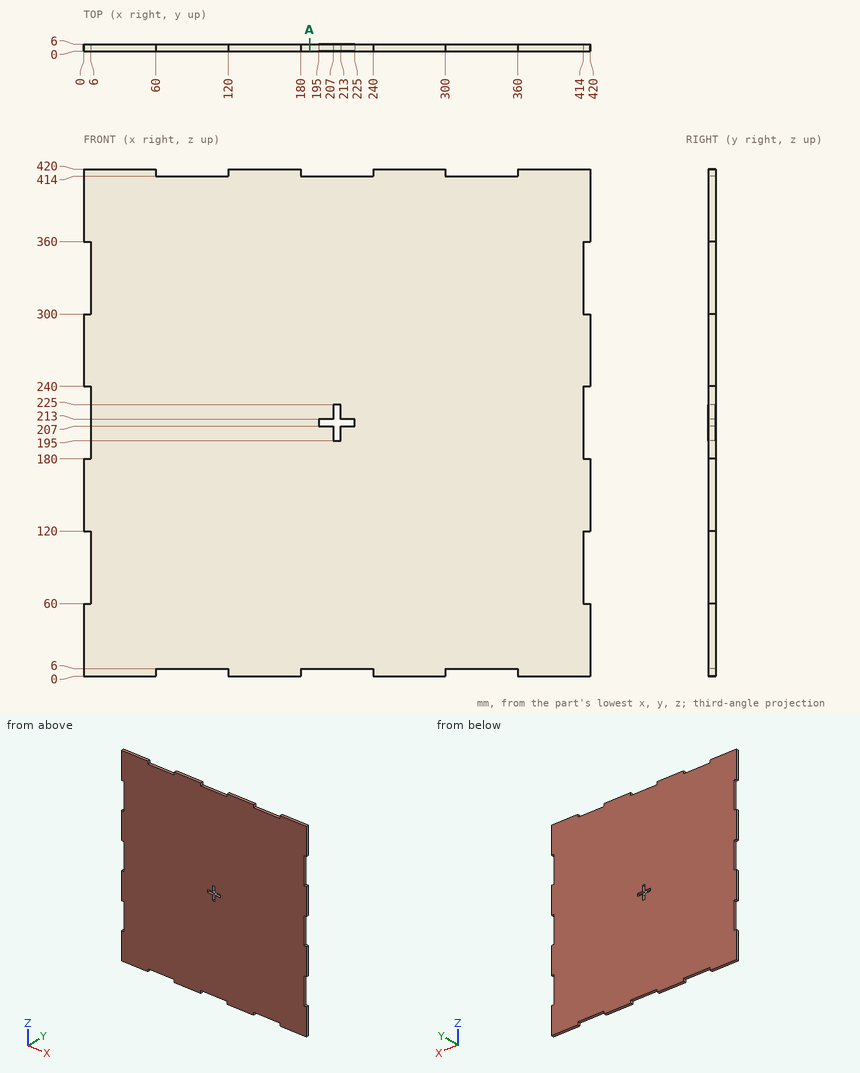
Input: dimensioned drawing with shaded views. Units: mm. Origin: part minimum x, y, z. Coordinates: 2 decimals unless noted, no trailing zeros. Order: outer loops, then holes, each group sorted by start corner. A loop starts at its lowest first (then second) coordinate and runs counter-clockwise, first axis right, second up.
1. Ray query, line 1 along X through (y, z) = (3, 212.5); line 2 along Z through (x, y) = (235, 4.6). Return the intervals inside material, ascending.
Checked values:
line 1: x = 6 to 195, 225 to 414
line 2: z = 6 to 414
2. Cut plane A-A, the plane x = 187.5. Return loops of the section in (y, z).
Checked values:
outline: (0, 6) - (6, 6) - (6, 414) - (0, 414) - close
3. Contact query for flat-ended pins moving along their axis: P1, Ø1.8, axis at y = 2, z = 201.5, coming from the -X side; P2, Ø3, axis at x = 329.5, y = 1.5, coming from the -Z side; P3, Ø1.8, axis at x = 195.5, y = 3.5, coming from the +Z side; P4, Ø1, axis at x = 132.5, y = 4, coming from the -Z side. Output: stop coordinate, or through.
Checked values:
P1: stops at x = 6
P2: stops at z = 6
P3: stops at z = 414
P4: stops at z = 0
